from build123d import *

# Parameters (mm, degrees)
SKETCH1_R                = 38
BOSS_EXTRUDE1_DEPTH      = 80
SKETCH2_R                = 29
CUT_EXTRUDE1_DEPTH       = 75
BOSS_EXTRUDE2_DEPTH      = 20
ESBO_O1_W                = 76
ESBO_O1_H                = 80
CORTE_EXTRUS_O1_DEPTH    = 155.518607294
ESBO_O2_W                = 2.5
ESBO_O2_H                = 49
RESSALTO_EXTRUS_O1_DEPTH = 5.4
ESBO_O3_R                = 1.35
CORTE_EXTRUS_O2_DEPTH    = 147.505972574
FILETE1_R                = 2


with BuildPart() as part:
    # Sketch1 → Boss-Extrude1 (new body)
    with BuildSketch(Plane(origin=(0, 0, 0), x_dir=(1, 0, 0), z_dir=(0, 1, 0))):
        with Locations(Location((0, 0, 0), (0, 0, 270))):
            Circle(SKETCH1_R)
    extrude(amount=BOSS_EXTRUDE1_DEPTH)

    # Sketch2 → Cut-Extrude1 (cut)
    with BuildSketch(Plane.XZ):
        with Locations(Location((0, 0, 0), (0, 0, 270))):
            Circle(SKETCH2_R)
    extrude(amount=-CUT_EXTRUDE1_DEPTH, mode=Mode.SUBTRACT)

    # Sketch3 → Boss-Extrude2 (add)
    with BuildSketch(Plane(origin=(0, 80, 0), x_dir=(1, 0, 0), z_dir=(0, 1, 0))):
        with BuildLine():
            Line((18, -90), (-18, -90))
            ThreePointArc((-18, -90), (-32.142135624, -84.142135624), (-38, -70))
            Line((-38, -70), (-38, 70))
            ThreePointArc((-38, 70), (-32.142135624, 84.142135624), (-18, 90))
            Line((-18, 90), (18, 90))
            ThreePointArc((18, 90), (32.142135624, 84.142135624), (38, 70))
            Line((38, 70), (38, -70))
            ThreePointArc((38, -70), (32.142135624, -84.142135624), (18, -90))
        make_face()
    extrude(amount=BOSS_EXTRUDE2_DEPTH)

    # Esboço1 → Corte-extrusão1 (cut, through all)
    with BuildSketch(Plane(origin=(38, 0, 0), x_dir=(0, 0, -1), z_dir=(1, 0, 0))):
        with Locations((0, 40)):
            Rectangle(ESBO_O1_W, ESBO_O1_H)
    extrude(amount=-CORTE_EXTRUS_O1_DEPTH, mode=Mode.SUBTRACT)

    # Esboço2 → Ressalto-extrusão1 (add)
    with BuildSketch(Plane.XZ.offset(-80)):
        with Locations((18.75, 0)):
            Rectangle(ESBO_O2_W, ESBO_O2_H)
        with Locations((-18.75, 0)):
            Rectangle(ESBO_O2_W, ESBO_O2_H)
    extrude(amount=RESSALTO_EXTRUS_O1_DEPTH)

    # Esboço3 → Corte-extrusão2 (cut, through all)
    with BuildSketch(Plane(origin=(20, 0, 0), x_dir=(0, 0, -1), z_dir=(1, 0, 0))):
        with Locations((22, 77.3)):
            Circle(ESBO_O3_R)
        with Locations((0, 77.3)):
            Circle(ESBO_O3_R)
        with Locations((-22, 77.3)):
            Circle(ESBO_O3_R)
    extrude(amount=-CORTE_EXTRUS_O2_DEPTH, mode=Mode.SUBTRACT)

    # Filete1
    filete1_edges = [part.edges().sort_by_distance(p)[0] for p in [
        (18.75, 74.6, -24.5),
        (18.75, 74.6, 24.5),
        (-18.75, 74.6, -24.5),
        (-18.75, 74.6, 24.5),
    ]]
    fillet(filete1_edges, radius=FILETE1_R)


solid = part.part
For this review, take the finished solid that the model builds, in its own axes (mm). A direction names the side the tool comes from. Coordinates: 2 decimals unless noted, no trailing zeros. Order: outer loops, then holes, each group sorted by start corner. A loop starts at its lowest first (then second) coordinate and runs counter-clockwise, first axis right, second up. Notation, with made-up numbers: (-36, 41.25) - (-8, 41.25) arc R29 cw to (-8, 69.25) - close; hole circle Ø5 at (60.5, 41.25). An arc over 180 degrees is marked (long way). Use one line per item in the form item = value.
Q1. Draft analysis for pull direction X (two halves, no side actions). For faces 1 (the cylindrical face through (-32.297, 89.86, -83.986)), 2 (the flat face through (17.5, 79, 0)), 3 (the flat face through (1, 80, -1)), 4 (the flat face through (0, 90, -90)), state which applies: +X half, -X half, draft (parallel to the pull), parting line (faces both ways), or undercut.
Checked values:
face_1 = -X half
face_2 = undercut
face_3 = undercut
face_4 = draft
Q2. For probe 1 along Z at (x, y) = (-19.2, 77.3); probe 2 along Y at (x, z) = (-19.15, -22); probe 3 along X at (y, z) = (78.5, -16.5), list the stretches that pass through material, from the lowest coordinate up. Write a range as from..to.
Checked values:
probe_1 = -24.5..-23.35, -20.65..-1.35, 1.35..20.65, 23.35..24.5
probe_2 = 74.6..75.95, 78.65..100
probe_3 = -20..-17.5, 17.5..20
Q3. Consider section A-A (z = -6). Give the boundary of the cut face in (x, y), then the cut area to 3 significant figures.
Checked values:
outline = (-38, 80) - (-20, 80) - (-20, 74.6) - (-17.5, 74.6) - (-17.5, 80) - (17.5, 80) - (17.5, 74.6) - (20, 74.6) - (20, 80) - (38, 80) - (38, 100) - (-38, 100) - close
area = 1,550 mm2
Q4. For faces 5 (the flat face through (-17.5, 79, 0)), 6 (the flat face through (-20, 79, 0)), 7 (the flat face through (20, 79, 0)), list the 3-axis set-ups (+Z, -Z, +X, -X, +Y, -Y) from which the entire face can be reached by the end or side of a thin tool; tool diameter is ignored.
Checked values:
face_5 = +Z, -Z, -Y
face_6 = +Z, -Z, -X, -Y
face_7 = +Z, -Z, +X, -Y
Q5. Consider section D-D (z = 63). Give the boundary of the cut face in (x, y).
Checked values:
outline = (-38, 80) - (38, 80) - (38, 100) - (-38, 100) - close
Q6. Consider section B-B (y = 97). Give the boundary of the cut face in (x, z).
Checked values:
outline = (-38, -70) arc R20 ccw to (-18, -90) - (18, -90) arc R20 ccw to (38, -70) - (38, 70) arc R20 ccw to (18, 90) - (-18, 90) arc R20 ccw to (-38, 70) - close
Q7. For P1, Ø2.5, axis at y = 77.3, z = -22, coming from the +X side; P2, Ø3, axis at x = -19, y = 78, coming from the -Z side; P3, Ø3, axis at y = 77.3, z = 22, coming from the -X side; P4, Ø2.5, axis at y = 78, z = -12, coming from the +X side, all flat-tipped, find the tip position at first contact; note any pin that passes through.
Checked values:
P1 = through
P2 = -24.5
P3 = -20
P4 = 20
Q8. Consider section C-C (x = -32.5). Give the boundary of the cut face in (y, z).
Checked values:
outline = (80, -83.77) - (100, -83.77) - (100, 83.77) - (80, 83.77) - close
